Autodesk Inventor part; units mm, degrees
ref_plane "YZ Plane" through (0, 0, 0) normal (1, 0, 0) x (0, 1, 0)
ref_plane "XZ Plane" through (0, 0, 0) normal (0, 1, 0) x (-1, 0, 0)
ref_plane "XY Plane" through (0, 0, 0) normal (0, 0, 1) x (1, 0, 0)
sketch "Sketch1" plane through (0, 0, 0) normal (0, 0, 1) x (1, 0, 0)
  line L0 (0, 0) -> (8.5, 0)
  line L1 (8.5, 0) -> (8.5, 6)
  line L2 (8.5, 6) -> (0, 6)
  line L3 (0, 6) -> (0, 0) construction
  circle A0 centre (0, 3) radius 3
  circle A1 centre (0, 3) radius 1.5
  dimension "d0" = 8.5
  dimension "d1" = 6
  dimension "d2" = 3
extrude "Extrusion1" add sketch "Sketch1" against normal blind 4.5
sketch "Sketch2" plane through (0, 6, 0) normal (0, 1, 0) x (1, 0, 0)
  line L0 (8.5, 0) -> (8.5, 4.5)
  line L1 (0, 0) -> (0, 0)
  line L2 (0, 0) -> (0, 4.5)
  line L3 (0, 4.5) -> (0, 4.5)
  line L4 (0, 0) -> (0, 4.5)
  line L5 (-3, 0) -> (-3, 4.5)
  line L6 (-3, 0) -> (0, 0)
  line L7 (0, 4.5) -> (-3, 4.5)
  line L8 (-3, 1.5) -> (4, 1.5)
  line L9 (4, 1.5) -> (4, 3)
  line L10 (4, 3) -> (-3, 3)
  line L11 (-3, 3) -> (-3, 1.5)
  point P0 (4, 2.25)
  point P1 (8.5, 2.25)
  dimension "d7" = 1.5
  dimension "d8" = 7
extrude "Extrusion2" cut sketch "Sketch2" against normal through all contours L8 L5 L10 L2 | L2 L10 L9 L8
sketch "Sketch3" plane through (8.5, 0, 0) normal (1, 0, 0) x (0, 0, -1)
  line L0 (4.5, 6) -> (4.5, 0)
  line L1 (0, 6) -> (4.5, 6)
  point P0 (2.25, 3)
  dimension "d11" = 3
  dimension "d12" = 2.25
hole "Hole1" at (8.5, 3, -2.25) direction (-1, 0, 0) diameter 2.459 depth 5.5 tip angle 118
properties part number "30 - Eccentric Rod 2" material "Steel AISI 1020 107 HR"
Build history of the part. All positions in model axes, mm. A direction names the side the tool comes from. Coordinates: 2 decimals unless noted, no trailing zeros. Order: outer loops, then holes, each group sorted by start corner. A loop starts at its lowest first (then second) coordinate and runs counter-clockwise, first axis right, second up.
Item 1: Tool access for faces 4 (the cylindrical face through (-3, 3, -4)), 5 (the cylindrical face through (5.71, 2.95, -1.02)), 6 (the flat face through (2, 3, -1.5)): list every direction of +Z, -Z, +X, -X, +Y, -Y with a clear straight run to the whole face (end or side of a thin tool).
Filled in:
face 4: +Z, -Z, -X
face 5: +X
face 6: -X, +Y, -Y
Item 2: Saw through at C-C on x = 2. List the corners of the cut face in (y, z).
Filled in:
outline: (0, -4.5) - (6, -4.5) - (6, -3) - (0, -3) - close; (0, -1.5) - (6, -1.5) - (6, 0) - (0, 0) - close
Item 3: Mould opens along Z. For faces 1 (the flat face through (4, 5, -2)), 2 (the flat face through (4, 3, -4.5)), 3 (the cylindrical face through (-0.325, 1.536, -3.74)) say: released by +Z, released by -Z, zero draft, split by the parting line, or undercut.
Filled in:
face 1: undercut
face 2: released by -Z
face 3: zero draft
Item 4: Saw through at A-A on y = 3. List the corners of the cut face in (x, z), then the cut area to 3 significant figures.
Filled in:
outline: (-3, -4.5) - (-1.5, -4.5) - (-1.5, -3) - (-3, -3) - close; (-3, -1.5) - (-1.5, -1.5) - (-1.5, 0) - (-3, 0) - close; (1.5, -4.5) - (8.5, -4.5) - (8.5, -3.48) - (3, -3.48) - (2.71, -3) - (1.5, -3) - close; (1.5, -1.5) - (2.71, -1.5) - (3, -1.02) - (8.5, -1.02) - (8.5, 0) - (1.5, 0) - close
area: 20.1 mm2
Item 5: Drill centre lines: L1, parallel to Y at x = 0, z = -3.8; L2, parallel to Z at x = 2.75, y = 1.4; L3, parallel to Z at x = 5.8, y = 3. Where is each one in solid material? Low to high.
Filled in:
L1: y = 0 to 1.5, 4.5 to 6
L2: z = -4.5 to -3, -1.5 to 0
L3: z = -4.5 to -3.48, -1.02 to 0
Item 6: Saw through at B-B on z = -4.15. List the corners of the cut face in (x, y).
Filled in:
outline: (0, 0) - (8.5, 0) - (8.5, 6) - (0, 6) arc R3 ccw to start; hole circle Ø3 at (0, 3)
Item 7: Saw through at D-D on z = -2.25. List the corners of the cut face in (x, y).
Filled in:
outline: (4, 0) - (8.5, 0) - (8.5, 1.77) - (4, 1.77) - close; (4, 4.23) - (8.5, 4.23) - (8.5, 6) - (4, 6) - close
Item 8: Drop flat-ended pins along their axis: pin 1 Ø2.5 at (x, y) = (0, 3) entering from +Z; pin 2 Ø1.5 at (x, z) = (-1.5, -2) entering from +Y; pin 3 Ø1.2 at (y, z) = (1.5, -2.5) entering from -X. Give the stop position or say it passes through.
Filled in:
pin 1: passes through
pin 2: stops at y = 5.85
pin 3: stops at x = -2.76
